Design review of the part built by this model. Coordinates are the model's own, in mm. Round coordinates to 2 decimals unless told otherwise and drop trailing zeros. Write each loop counter-clockwise with the first axis right and the second up, starting at its lowest first coordinate (ties: lowest second). Pieces come first, ordered by that corner, then holes. Notation, with made-up numbers: (77.25, 1.5) -> (82.25, 1.5) arc R19 cw to (82.25, 38.5) -> close; hole circle Ø9 at (4, 78). An arc over 180 degrees is marked (long way). One line per question, with ' | ' between items. Start each with the question number.
1) Consider section A-A (z = 0). Give the boundary of the cut face in (x, y), then the cut area to 3 significant figures.
2) Consider section D-D (x = 7.5). Give the boundary of the cut face in (y, z).
3) Mouldability with a two-part tool opening along Y and no side actions: class faces 1 (the flat face through (10, 0, 0)), 2 (the conical face through (10.01, -5.02, 15.95)), 3 (the flat face through (0, 0, 0)) as +Y half, -Y half, draft (parallel to the pull), parting line (faces both ways), or undercut.
4) Insertion check: pin 1 Ø1 at (x, z) = (44.5, -13.5) entering from -Y; pin 2 Ø1.5 at (x, y) = (47.5, -11) entering from +Z; pin 3 Ø5 at (x, z) = (57.5, -10) entering from +Y. Each pin has a flat end and moves straight along its axis. Give the tip position at first contact, or say it passes through.
5) Consider section C-C (x = 23.5). Give the boundary of the cut face in (y, z).
6) For probe 1 along Y at (x, z) = (6.5, 0); probe 2 along Z at (x, y) = (54.5, -3); probe 3 along X at (y, z) = (3, -2), list the stretches that pass through material, from the lowest coordinate up.
```python
from build123d import *

# Parameters (mm, degrees)
SKETCH6_R           = 13
BOSS_EXTRUDE1_DEPTH = 10
SKETCH7_R           = 1.5
CUT_EXTRUDE1_DEPTH  = 10


with BuildPart() as part:
    # Sketch2 → Revolve5 (revolve)
    with BuildSketch(Plane.XY, mode=Mode.PRIVATE) as revolve5_sk:
        Polygon((0, 13), (0, 7.888355817), (80, 24.888355817), (80, 30), (36.968539733, 26.749080476), align=None)
    revolve(revolve5_sk.sketch.rotate(Axis((0, 0, 0), (1, 0, 0)), 90), axis=Axis((0, 0, 0), (1, 0, 0)))

    # Sketch6 → Boss-Extrude1 (add)
    with BuildSketch(Plane.ZY):
        Circle(SKETCH6_R)
    extrude(amount=-BOSS_EXTRUDE1_DEPTH)

    # Sketch7 → Cut-Extrude1 (cut)
    with BuildSketch(Plane.ZY):
        with Locations((0, 8)):
            Circle(SKETCH7_R)
        with Locations((0, -8)):
            Circle(SKETCH7_R)
        with Locations((8, 0)):
            Circle(SKETCH7_R)
        with Locations((-8, 0)):
            Circle(SKETCH7_R)
    extrude(amount=-CUT_EXTRUDE1_DEPTH, mode=Mode.SUBTRACT)


solid = part.part
```
From the geometry:
1) outline: (0, -13) -> (36.97, -26.75) -> (80, -30) -> (80, -24.89) -> (10, -10.01) -> (10, -9.5) -> (0, -9.5) -> close; (0, -6.5) -> (10, -6.5) -> (10, 6.5) -> (0, 6.5) -> close; (0, 9.5) -> (10, 9.5) -> (10, 10.01) -> (80, 24.89) -> (80, 30) -> (36.97, 26.75) -> (0, 13) -> close | area: 1,410 mm2
2) outline: circle Ø31.58 at (0, 0); hole circle Ø3 at (-8, 0); hole circle Ø3 at (0, -8); hole circle Ø3 at (0, 8); hole circle Ø3 at (8, 0)
3) face 1: undercut | face 2: parting line | face 3: draft
4) pin 1: stops at y = -24.03 | pin 2: stops at z = 25.57 | pin 3: stops at y = 27.32
5) outline: circle Ø43.48 at (0, 0); hole circle Ø25.76 at (0, 0)
6) probe 1: y = -15.42 to -9.5, -6.5 to 6.5, 9.5 to 15.42 | probe 2: z = -27.91 to -19.24, 19.24 to 27.91 | probe 3: x = 0 to 10
